Part model, mm, in its own coordinate system. Face numbers are marked on the shaded views. Round coordinates to 2 decimals unless told otherwise and drop trailing zeros. Order: outer loops, then holes, each group sorted by start corner. A loop starts at its lowest first (then second) coordinate and runs counter-clockwise, first axis right, second up. Notation, with made-up numbers: (10.25, 35) -> (50.25, 35) arc R18 ccw to (50.25, 70) -> close; hole circle Ø7 at (6.5, 83). An arc over 180 degrees is marked (long way). Use CSV: the item, a comma, the result in double quotes.
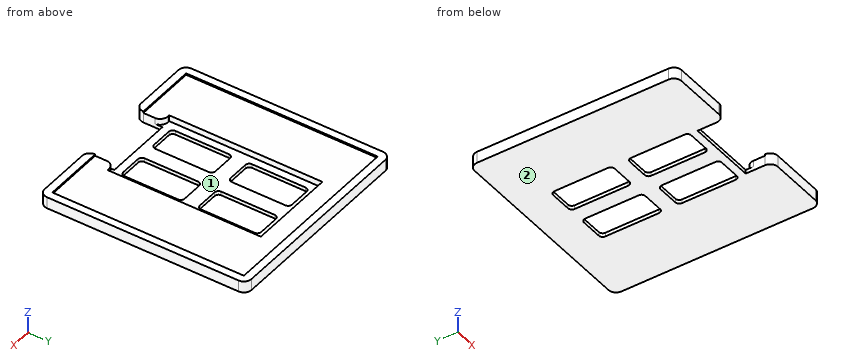
```python
from build123d import *

# Parameters (mm, degrees)
SKETCH_1_W          = 54
SKETCH_1_H          = 54
EXTRUDE_1_DEPTH     = 3
SKETCH_2_W          = 23
SKETCH_2_H          = 40
CUT_EXTRUDE_1_DEPTH = 2
SKETCH_3_W          = 50
SKETCH_3_H          = 50
CUT_EXTRUDE_2_DEPTH = 0.4
SKETCH_4_W          = 18
SKETCH_4_H          = 7
CUT_EXTRUDE_3_DEPTH = 39.301436004
SKETCH_5_W          = 7.5
SKETCH_5_H          = 16
CUT_EXTRUDE_4_DEPTH = 39.236108589
FILLET_1_R          = 2
FILLET_2_R          = 1
FILLET_3_R          = 2


with BuildPart() as part:
    # Эскиз1 → Бобышка-Вытянуть1 (new body)
    with BuildSketch(Plane.XY):
        Rectangle(SKETCH_1_W, SKETCH_1_H)
    extrude(amount=EXTRUDE_1_DEPTH)

    # Эскиз2 → Вырез-Вытянуть1 (cut)
    with BuildSketch(Plane.XY.offset(3)):
        Rectangle(SKETCH_2_W, SKETCH_2_H)
    extrude(amount=-CUT_EXTRUDE_1_DEPTH, mode=Mode.SUBTRACT)

    # Эскиз3 → Вырез-Вытянуть2 (cut)
    with BuildSketch(Plane.XY.offset(3)):
        Rectangle(SKETCH_3_W, SKETCH_3_H)
    extrude(amount=-CUT_EXTRUDE_2_DEPTH, mode=Mode.SUBTRACT)

    # Эскиз4 → Вырез-Вытянуть3 (cut, through all)
    with BuildSketch(Plane.XY.offset(3)):
        with Locations((0, -23.5)):
            Rectangle(SKETCH_4_W, SKETCH_4_H)
    extrude(amount=-CUT_EXTRUDE_3_DEPTH, mode=Mode.SUBTRACT)

    # Эскиз5 → Вырез-Вытянуть4 (cut, through all)
    with BuildSketch(Plane.XY.offset(1)):
        with Locations((-5.75, 10)):
            Rectangle(SKETCH_5_W, SKETCH_5_H)
        with Locations((5.75, 10)):
            Rectangle(SKETCH_5_W, SKETCH_5_H)
        with Locations((-5.75, -10)):
            Rectangle(SKETCH_5_W, SKETCH_5_H)
        with Locations((5.75, -10)):
            Rectangle(SKETCH_5_W, SKETCH_5_H)
    extrude(amount=-CUT_EXTRUDE_4_DEPTH, mode=Mode.SUBTRACT)

    # Скругление1
    fillet_1_edges = [part.edges().sort_by_distance(p)[0] for p in [
        (9, -27, 1.5),
        (9, -20, 1.8),
        (-9, -27, 1.5),
        (-9, -20, 1.8),
    ]]
    fillet(fillet_1_edges, radius=FILLET_1_R)

    # Скругление2
    fillet_2_edges = [part.edges().sort_by_distance(p)[0] for p in [
        (2, -18, 0.5),
        (2, -2, 0.5),
        (9.5, -2, 0.5),
        (9.5, -18, 0.5),
        (-2, 18, 0.5),
        (-2, 2, 0.5),
        (-9.5, 2, 0.5),
        (-9.5, 18, 0.5),
        (9.5, 2, 0.5),
        (2, 2, 0.5),
        (2, 18, 0.5),
        (9.5, 18, 0.5),
        (-9.5, -2, 0.5),
        (-2, -2, 0.5),
        (-2, -18, 0.5),
        (-9.5, -18, 0.5),
    ]]
    fillet(fillet_2_edges, radius=FILLET_2_R)

    # Скругление3
    fillet_3_edges = [part.edges().sort_by_distance(p)[0] for p in [
        (27, -27, 1.5),
        (-27, -27, 1.5),
        (-27, 27, 1.5),
        (27, 27, 1.5),
    ]]
    fillet(fillet_3_edges, radius=FILLET_3_R)


solid = part.part
```
(1) Pull direction Y, two halves, no side cores. Call the marked faces 1 and 2: released by +Y, released by -Y, zero draft, split by the parting line, or undercut.
Reply:
face 1,"undercut"
face 2,"zero draft"
(2) Cut at A-A, the plane y = 5. Give the cut face in (x, z).
Reply:
outline,"(-27, 0) -> (-9.5, 0) -> (-9.5, 1) -> (-11.5, 1) -> (-11.5, 2.6) -> (-25, 2.6) -> (-25, 3) -> (-27, 3) -> close; (-2, 0) -> (2, 0) -> (2, 1) -> (-2, 1) -> close; (9.5, 0) -> (27, 0) -> (27, 3) -> (25, 3) -> (25, 2.6) -> (11.5, 2.6) -> (11.5, 1) -> (9.5, 1) -> close"
(3) Cut at B-B, the plane x = -5.5. Give the cut face in (y, z), then the cut area to 3 significant figures.
Reply:
outline,"(-20, 0) -> (-18, 0) -> (-18, 1) -> (-20, 1) -> close; (-2, 0) -> (2, 0) -> (2, 1) -> (-2, 1) -> close; (18, 0) -> (27, 0) -> (27, 3) -> (25, 3) -> (25, 2.6) -> (20, 2.6) -> (20, 1) -> (18, 1) -> close"
area,"27.0 mm2"
(4) Drop flat-ended pins along their axis: P1, Ø0.5, axis at x = -7, z = 0.5, coming from the -Y side; P2, Ø4, axis at x = 3, y = 18.5, coming from the -Z side; P3, Ø8, axis at x = -18.5, y = 0.5, coming from the +Z side; P4, Ø0.5, axis at x = 4, z = 2, coming from the -Y side. Give the stop position or say it passes through.
Reply:
P1,"y = -20"
P2,"z = 0"
P3,"z = 2.6"
P4,"y = 20"
(5) Probe probe 1 along X at (y, z) = (-8, 0.7); probe 2 along Y at (x, z) = (-3, 0.75); probe 3 along X at (y, z) = (7.5, 1.4). List the from-to ranges inside material, lowest first. Write a range as [from, to].
Reply:
probe 1,"[-27, -9.5], [-2, 2], [9.5, 27]"
probe 2,"[-20, -18], [-2, 2], [18, 27]"
probe 3,"[-27, -11.5], [11.5, 27]"
(6) Cut at D-D, the plane z = 1.6. Give the cut face in (x, y).
Reply:
outline,"(-27, -25) arc R2 ccw to (-25, -27) -> (-11, -27) arc R2 ccw to (-9, -25) -> (-9, -22) arc R2 ccw to (-11, -20) -> (-11.5, -20) -> (-11.5, 20) -> (11.5, 20) -> (11.5, -20) -> (11, -20) arc R2 ccw to (9, -22) -> (9, -25) arc R2 ccw to (11, -27) -> (25, -27) arc R2 ccw to (27, -25) -> (27, 25) arc R2 ccw to (25, 27) -> (-25, 27) arc R2 ccw to (-27, 25) -> close"
(7) Cut at C-C, the plane x = 0. Give the cut face in (y, z).
Reply:
outline,"(-20, 0) -> (27, 0) -> (27, 3) -> (25, 3) -> (25, 2.6) -> (20, 2.6) -> (20, 1) -> (-20, 1) -> close"
